from build123d import *

# Parameters (mm, degrees)
EXTRUDE1_DEPTH = 6.35
SKETCH3_R      = 1.5875
EXTRUDE2_DEPTH = 12.7
SKETCH4_R      = 1.5875
EXTRUDE3_DEPTH = 12.7
SKETCH6_W      = 19.05
SKETCH6_H      = 0.635
EXTRUDE4_DEPTH = 6.35
SKETCH8_R      = 6.35
EXTRUDE5_DEPTH = 6.35


with BuildPart() as part:
    # Sketch1 → Extrude1 (new body)
    with BuildSketch(Plane.XY):
        Polygon((-15.437909459, 32.870050856), (-15.437909459, -93.380203425), (61.751637834, -93.380203425), (80.801637834, -93.380203425), (80.801637834, -67.980203425), (61.751637834, -67.980203425), align=None)
    extrude(amount=EXTRUDE1_DEPTH)

    # Sketch3 → Extrude2 (cut)
    with BuildSketch(Plane.XZ.offset(93.380203425)):
        with Locations(Location((-8.098362166, 3.175, 0), (0, 0, 270))):
            Circle(SKETCH3_R)
        with Locations(Location((68.101637834, 3.175, 0), (0, 0, 270))):
            Circle(SKETCH3_R)
    extrude(amount=-EXTRUDE2_DEPTH, mode=Mode.SUBTRACT)

    # Sketch4 → Extrude3 (cut)
    with BuildSketch(Plane(origin=(6.12959486, 4.691516702, 0), x_dir=(0, 0, -1), z_dir=(0.7940964904073088, 0.6077917109691402, 0))):
        with Locations(Location((-3.175, 10.085025428, 0), (0, 0, 90))):
            Circle(SKETCH4_R)
    extrude(amount=-EXTRUDE3_DEPTH, mode=Mode.SUBTRACT)

    # Sketch6 → Extrude4 (cut)
    with BuildSketch(Plane(origin=(0, -67.980203425, 0), x_dir=(1, 0, 0), z_dir=(0, 1, 0))):
        with Locations((71.276637834, -3.4925)):
            Rectangle(SKETCH6_W, SKETCH6_H)
    extrude(amount=-EXTRUDE4_DEPTH, mode=Mode.SUBTRACT)

    # Sketch8 → Extrude5 (cut)
    with BuildSketch(Plane(origin=(6.12959486, 4.691516702, 0), x_dir=(0, 0, -1), z_dir=(0.7940964904073088, 0.6077917109691404, 0))):
        with Locations((-3.175, 10.085025428)):
            Circle(SKETCH8_R)
    extrude(amount=-EXTRUDE5_DEPTH, mode=Mode.SUBTRACT)


solid = part.part
Input: part model. Units: mm. Frame: model coordinates. A direction names the side the tool comes from. Give positions to 0.01 mm unless a question says otherwise; leave off trailing zeros. Loops run counter-clockwise (first coordinate to the right, second up) from the corner with the lowest first, then second, coordinate; pieces in that order, holes last. Notation, with made-up numbers: (13, -28.5) -> (23, -28.5) arc R26 ccw to (23, 0.5) -> close; hole circle Ø5 at (57.25, -39.75). An arc over 180 degrees is marked (long way). Answer as a JSON object with one key per item and string values. Group by question number.
Item 1: Pin query (flat end, axial travel): P1, Ø1, axis at y = 9.5, z = 5.5, coming from the +X side; P2, Ø0.5, axis at x = 75, z = 3.5, coming from the +Y side; P3, Ø1.5, axis at y = 6, z = 4.5, coming from the +X side. Return the tip coordinate at first contact, or that it passes through.
Item 2: Reachability of faces 1 (the flat face through (-4.24, 7.79, 1.81)), 2 (the cylindrical face through (-9.507, -87.119, 2.442)), 3 (the cylindrical face through (1.37, 5.75, 3.22)), 4 (the flat face through (71, -71, 3.81)), 5 (the cylindrical face through (-6.345, 15.84, 3.128)) from +Z, -Z, +X, -X, +Y, -Y: full face, straight path, thin tool, end or side. Return the list, or none.
Item 3: Cut plane B-B, the plane x = 73. Return the cut outline in (y, z) (3 decimals).
Item 4: Cut plane D-D, the plane y = -26.5. Return the cut outline in (x, z), and give its area (3 significant figures).
Item 5: Cut plane A-A, the plane y = -72. Return the cut outline in (x, z) (3 decimals), and give its area (3 significant figures).
Item 6: Pull-direction query (Y, two-part tool) for faces 6 (the flat face through (71, -67.98, 2)), 7 (the cylindrical face through (66.552, -87.119, 3.519)), 8 (the flat face through (-10.1, 5, 3.2)); classes: released by +Y, released by -Y, zero draft, split by the parting line, or undercut.
Item 7: Cut plane C-C, the plane x = 8.5. Return the cut outline in (y, z).
Item 8: Line query: probe 1 along Y at (x, z) = (40, 2.25); probe 2 along Y at (x, z) = (37, 4.5); probe 3 along X at (y, z) = (21.5, 2.25). Output: solid intervals per line, ascending.
Checks:
{
 "1": {"P1": "stops at x = -5.16", "P2": "stops at y = -74.33", "P3": "stops at x = 5.7"},
 "2": {"face 1": "none", "face 2": "-Y", "face 3": "+Y", "face 4": "+X, +Y", "face 5": "+X"},
 "3": {"outline": "(-93.38, 0) -> (-67.98, 0) -> (-67.98, 3.175) -> (-74.33, 3.175) -> (-74.33, 3.81) -> (-67.98, 3.81) -> (-67.98, 6.35) -> (-93.38, 6.35) -> close"},
 "4": {"outline": "(-15.44, 0) -> (30, 0) -> (30, 6.35) -> (-15.44, 6.35) -> close", "area": "289 mm²"},
 "5": {"outline": "(-15.438, 0) -> (80.802, 0) -> (80.802, 3.175) -> (61.752, 3.175) -> (61.752, 3.81) -> (80.802, 3.81) -> (80.802, 6.35) -> (-15.438, 6.35) -> close", "area": "599 mm²"},
 "6": {"face 6": "released by +Y", "face 7": "zero draft", "face 8": "undercut"},
 "7": {"outline": "(-93.38, 0) -> (1.59, 0) -> (1.59, 6.35) -> (-93.38, 6.35) -> close"},
 "8": {"probe 1": "y = -93.38 to -39.56", "probe 2": "y = -93.38 to -35.64", "probe 3": "x = -15.44 to -6.74"}
}
